The listing builds one solid part. Answer for the finished solid, in the listing's coordinates (mm). Face numbers are marked on the shaded views. A direction names the side the tool comes from. Coordinates: 2 decimals unless noted, no trailing zeros. Order: outer loops, then holes, each group sorted by start corner. A loop starts at its lowest first (then second) coordinate and runs counter-clockwise, first axis right, second up.
from build123d import *

# Parameters (mm, degrees)
F0_W           = 140
F0_H           = 140
F0_R           = 42.5
F1_DEPTH       = 95
F2_R           = 47.5
F2_R_2         = 42.5
F3_DEPTH       = 3
F4_R           = 47.5
F4_R_2         = 42.5
F5_DEPTH       = 3
F8_DEPTH       = 98.001
F9_D           = 6
F9_CBORE_D     = 20
F9_CBORE_DEPTH = 30


with BuildPart() as f1:
    # F0 (on Top) → F1 (new body)
    with BuildSketch(Plane.XY):
        Rectangle(F0_W, F0_H)
        Circle(F0_R, mode=Mode.SUBTRACT)
    extrude(amount=F1_DEPTH)

    # F2 (on face) → F3 (join)
    with BuildSketch(Plane.XY.offset(95)):
        Circle(F2_R)
        Circle(F2_R_2, mode=Mode.SUBTRACT)
    extrude(amount=F3_DEPTH)

    # F4 (on face) → F5 (cut)
    with BuildSketch(Plane(origin=(0, 0, 0), x_dir=(1, 0, 0), z_dir=(0, 0, -1))):
        Circle(F4_R)
        Circle(F4_R_2, mode=Mode.SUBTRACT)
    extrude(amount=-F5_DEPTH, mode=Mode.SUBTRACT)

    # F7 (on face) → F8 (cut, through all)
    with BuildSketch(Plane(origin=(0, 0, 0), x_dir=(1, 0, 0), z_dir=(0, 0, -1))):
        with BuildLine():
            ThreePointArc((-62.5, 0), (-60.957820374, -3.6115755926), (-57.2826086957, -4.9952718666))
            ThreePointArc((-57.2826086957, -4.9952718666), (-57.4456264654, -2.5), (-57.5, 0))
            Line((-57.5, 0), (-62.5, 0))
        make_face()
        with BuildLine():
            ThreePointArc((-57.5, 0), (-57.4456264654, -2.5), (-57.2826086957, -4.9952718666))
            ThreePointArc((-57.2826086957, -4.9952718666), (-53.8884244074, -3.457820374), (-52.5, 0))
            Line((-52.5, 0), (-57.5, 0))
        make_face()
        with BuildLine():
            ThreePointArc((-52.5, 0), (-53.8884244074, 3.457820374), (-57.2826086957, 4.9952718666))
            ThreePointArc((-57.2826086957, 4.9952718666), (-57.4456264654, 2.5), (-57.5, 0))
            Line((-57.5, 0), (-52.5, 0))
        make_face()
        with BuildLine():
            ThreePointArc((-57.5, 0), (-57.4456264654, 2.5), (-57.2826086957, 4.9952718666))
            ThreePointArc((-57.2826086957, 4.9952718666), (-60.957820374, 3.6115755926), (-62.5, 0))
            Line((-62.5, 0), (-57.5, 0))
        make_face()
        with BuildLine():
            ThreePointArc((-4.9952718666, -57.2826086957), (0, -57.5), (4.9952718666, -57.2826086957))
            ThreePointArc((4.9952718666, -57.2826086957), (0, -52.5), (-4.9952718666, -57.2826086957))
        make_face()
        with BuildLine():
            ThreePointArc((5, -57.5), (4.9988178269, -57.3912786423), (4.9952718666, -57.2826086957))
            ThreePointArc((4.9952718666, -57.2826086957), (0, -57.5), (-4.9952718666, -57.2826086957))
            ThreePointArc((-4.9952718666, -57.2826086957), (-0.1087213577, -62.4988178269), (5, -57.5))
        make_face()
        with BuildLine():
            ThreePointArc((57.2826086957, 4.9952718666), (57.4456264654, 2.5), (57.5, 0))
            ThreePointArc((57.5, 0), (57.4456264654, -2.5), (57.2826086957, -4.9952718666))
            ThreePointArc((57.2826086957, -4.9952718666), (60.957820374, -3.6115755926), (62.5, 0))
            ThreePointArc((62.5, 0), (60.957820374, 3.6115755926), (57.2826086957, 4.9952718666))
        make_face()
        with BuildLine():
            ThreePointArc((57.2826086957, -4.9952718666), (57.4456264654, -2.5), (57.5, 0))
            ThreePointArc((57.5, 0), (57.4456264654, 2.5), (57.2826086957, 4.9952718666))
            ThreePointArc((57.2826086957, 4.9952718666), (52.5, 0), (57.2826086957, -4.9952718666))
        make_face()
        with BuildLine():
            ThreePointArc((-4.9952718666, 57.2826086957), (0, 52.5), (4.9952718666, 57.2826086957))
            ThreePointArc((4.9952718666, 57.2826086957), (0, 57.5), (-4.9952718666, 57.2826086957))
        make_face()
        with BuildLine():
            ThreePointArc((-4.9952718666, 57.2826086957), (0, 57.5), (4.9952718666, 57.2826086957))
            ThreePointArc((4.9952718666, 57.2826086957), (4.9988178269, 57.3912786423), (5, 57.5))
            ThreePointArc((5, 57.5), (-0.1087213577, 62.4988178269), (-4.9952718666, 57.2826086957))
        make_face()
    extrude(amount=-F8_DEPTH, mode=Mode.SUBTRACT)

    # F9 (through all)
    with Locations(Plane(origin=(0, 0, 0), x_dir=(1, 0, 0), z_dir=(0, 0, -1))):
        with Locations((-45.9619407771, -45.9619407771), (-45.9619407771, 45.9619407771), (45.9619407771, -45.9619407771), (45.9619407771, 45.9619407771)):
            CounterBoreHole(F9_D / 2, F9_CBORE_D / 2, F9_CBORE_DEPTH)


solid = f1.part
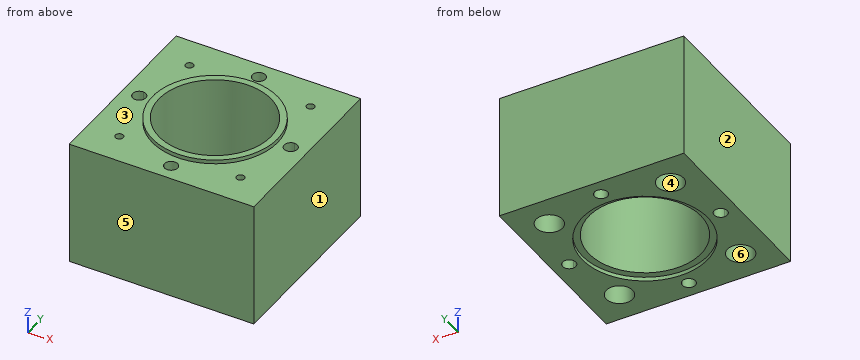
(1) Find section B-B on z = 73. Count the separate pieces of the cut face and the enclosed holes in it, then the cut area to 3 significant figures.
(2) Find section C-C on y = 7.5. Determine the outline of the cut face in (x, z), then the cut area to 3 significant figures.
(3) The mould has two halves that part along X. Classify the marked faces 1, 2, 3 and 4: pulls with the +X half, pulls with the -X half, needs draft (parallel to the pull), parting line crosses it, or undercut.
(4) A tool of negligible diameter and unlimited length cuts with its end or side. For the marked faces 5 and 6, from which of +Z, -Z, +X, -X, +Y, -Y can it reach the whole face along a straight path? Write none if from no direction.
(5) Find section A-A on x = 10.5. Determine the outline of the cut face in (y, z).
(6) Given pin 1 Ø3.5 at (x, y) = (-45.96, 45.96) entering from +Z (3 decimals); pin 2 Ø16 at (x, y) = (45.96, 45.96) entering from +Z; pin 3 Ø12 at (x, y) = (-45.96, -45.96) entering from -Z, each flat-ended and moving along its own axis, determine where each tip first touches the part or whether it passes through.
(7) Find the intervals of material crossed by probe 1 along Y at (x, z) = (-0.5, 11.5); probe 2 along Y at (x, z) = (-3, 73); probe 3 along Y at (x, z) = (-49, 24), in increasing order.
Resolved:
1. separate pieces: 1
1. enclosed holes: 9
1. area: 13,500 mm2
2. outline: (-70, 0) - (-46.9, 0) - (-46.9, 3) - (-41.83, 3) - (-41.83, 98) - (-46.9, 98) - (-46.9, 95) - (-70, 95) - close; (41.83, 3) - (46.9, 3) - (46.9, 0) - (70, 0) - (70, 95) - (46.9, 95) - (46.9, 98) - (41.83, 98) - close
2. area: 5,350 mm2
3. face 1: pulls with the +X half
3. face 2: pulls with the -X half
3. face 3: needs draft
3. face 4: undercut
4. face 5: +Z, -Z, +X, -X, -Y
4. face 6: -Z
5. outline: (-70, 0) - (-46.32, 0) - (-46.32, 3) - (-41.18, 3) - (-41.18, 98) - (-46.32, 98) - (-46.32, 95) - (-70, 95) - close; (41.18, 3) - (46.32, 3) - (46.32, 0) - (70, 0) - (70, 95) - (46.32, 95) - (46.32, 98) - (41.18, 98) - close
6. pin 1: passes through
6. pin 2: stops at z = 95
6. pin 3: stops at z = 30
7. probe 1: y = -70 to -62.47, -52.53 to -42.5, 42.5 to 52.53, 62.47 to 70
7. probe 2: y = -70 to -61.5, -53.5 to -42.39, 42.39 to 53.5, 61.5 to 70
7. probe 3: y = -70 to -55.49, -36.43 to 36.43, 55.49 to 70
